Geometry: final body of the model. Coordinates: model frame, mm. A direction names the side the tool comes from. Give positions to 0.01 mm unless a question says otherwise; leave off trailing zeros. Write each loop counter-clockwise with the first axis right and the second up, starting at its lowest first coordinate (ties: lowest second). Pieces come first, ordered by that corner, then holes.
Q1. Line query: line 1 (X direction, y = 6.5, z = 10.5); line 2 (Z direction, x = 18, y = 8.25); line 3 (X direction, y = 3, z = -28). Output: solid intervals per line, ascending.
Q2. Pin query (flat end, axial travel): pin 1 Ø2 at (x, y) = (37, 5) entering from -Z; pin 2 Ø3 at (y, z) = (7.5, -34) entering from +X. Return the tip coordinate at first contact, or that it passes through.
Q3. Reachability of faces 1 (the flat face through (37.1, 4.93, -34.85)), 2 (the flat face through (-35, 5, 32)), 3 (the cylindrical face through (34.84, 9.699, 32.563)), 4 (the cylindrical face through (35.063, 0.301, -32.34)) from +Z, -Z, +X, -X, +Y, -Y: full face, straight path, thin tool, end or side. Return the list, or none.
Q4. Section B-B (z = 13). Return the cut outline in (x, y), plus the area to 3 significant figures.
Q5. Section A-A (x = -10.5). Return the cut outline in (y, z), plus the area to 3 significant figures.
from build123d import *

# Parameters (mm, degrees)
BOSS_EXTRUDE1_DEPTH = 10
FILLET1_R           = 1


with BuildPart() as part:
    # Sketch1 → Boss-Extrude1 (new body)
    with BuildSketch(Plane(origin=(0, 0, 0), x_dir=(1, 0, 0), z_dir=(0, 1, 0))):
        Polygon((-46.5, 25.449747468), (-27.949747468, 44), (27.949747468, 44), (46.5, 25.449747468), (46.5, -25.449747468), (27.949747468, -44), (-27.949747468, -44), (-46.5, -25.449747468), align=None)
        Polygon((-43, 24), (-26.5, 40.5), (26.5, 40.5), (43, 24), (43, -24), (26.5, -40.5), (-26.5, -40.5), (-43, -24), align=None, mode=Mode.SUBTRACT)
    extrude(amount=BOSS_EXTRUDE1_DEPTH)

    # Fillet1
    fillet1_edges = [part.edges().sort_by_distance(p)[0] for p in [
        (-46.5, 5, -25.449747468),
        (-27.949747468, 5, -44),
        (27.949747468, 5, -44),
        (46.5, 5, -25.449747468),
        (46.5, 5, 25.449747468),
        (27.949747468, 5, 44),
        (-27.949747468, 5, 44),
        (-46.5, 5, 25.449747468),
        (-43, 0, 0),
        (-43, 5, -24),
        (-34.75, 0, 32.25),
        (-43, 5, 24),
        (0, 0, 40.5),
        (-26.5, 5, 40.5),
        (34.75, 0, 32.25),
        (26.5, 5, 40.5),
        (43, 0, 0),
        (43, 5, 24),
        (34.75, 0, -32.25),
        (43, 5, -24),
        (0, 0, -40.5),
        (26.5, 5, -40.5),
        (-34.75, 0, -32.25),
        (-26.5, 5, -40.5),
        (-43, 10, 0),
        (-34.75, 10, 32.25),
        (0, 10, 40.5),
        (34.75, 10, 32.25),
        (43, 10, 0),
        (34.75, 10, -32.25),
        (0, 10, -40.5),
        (-34.75, 10, -32.25),
    ]]
    fillet(fillet1_edges, radius=FILLET1_R)


solid = part.part
Computed:
1. line 1: x = -46.5 to -43, 43 to 46.5
1. line 2: z = -44 to -40.5, 40.5 to 44
1. line 3: x = -43.95 to -39, 39 to 43.95
2. pin 1: stops at z = -35.95
2. pin 2: stops at x = 39.45
3. face 1: -Z, +X, +Y, -Y
3. face 2: +Y, -Y
3. face 3: +Y
3. face 4: -Y
4. outline: (-46.5, 0) - (-44, 0) arc R1 ccw to (-43, 1) - (-43, 9) arc R1 ccw to (-44, 10) - (-46.5, 10) - close; (43, 1) arc R1 ccw to (44, 0) - (46.5, 0) - (46.5, 10) - (44, 10) arc R1 ccw to (43, 9) - close
4. area: 69.1 mm2
5. outline: (0, -44) - (10, -44) - (10, -41.5) arc R1 ccw to (9, -40.5) - (1, -40.5) arc R1 ccw to (0, -41.5) - close; (0, 41.5) arc R1 ccw to (1, 40.5) - (9, 40.5) arc R1 ccw to (10, 41.5) - (10, 44) - (0, 44) - close
5. area: 69.1 mm2
